Design review of the part built by this model. Coordinates are the model's own, in mm. A direction names the side the tool comes from. Round coordinates to 2 decimals unless told otherwise and drop trailing zeros. Order: outer loops, then holes, each group sorted by start corner. A loop starts at its lowest first (then second) coordinate and runs counter-clockwise, first axis right, second up. Notation, with made-up numbers: (74.5, -40) - (119.5, -40) arc R18 ccw to (119.5, -14) - close; hole circle Ø6 at (5, 77). An arc over 180 degrees is marked (long way). Answer as a JSON object with one key per item and string values. Group by question number.
from build123d import *

# Parameters (mm, degrees)
SKETCH3_W                      = 207
SKETCH3_H                      = 195
BASE_FLANGE1_DEPTH             = 2
EDGE_FLANGE1_STRIP_W           = 9.4732
EDGE_FLANGE1_STRIP_H           = 2
EDGE_FLANGE1_STRIP_CUT_DEPTH   = 207
EDGE_FLANGE1_STRIP_2_W         = 9.4732
EDGE_FLANGE1_STRIP_2_H         = 2
EDGE_FLANGE1_STRIP_CUT_2_DEPTH = 207
EDGE_FLANGE1_DEPTH             = 207
EDGE_FLANGE1_BEND_DEPTH        = 207
SKETCH14_R                     = 68.5
CUT_EXTRUDE1_DEPTH             = 2
EDGE_FLANGE2_DEPTH             = 207
EDGE_FLANGE2_BEND_DEPTH        = 207


# Sheet-metal steps are written as plain solids
with BuildPart() as part:
    # Sketch3 → Base-Flange1 (new body)
    with BuildSketch(Plane(origin=(0, 0, 0), x_dir=(1, 0, 0), z_dir=(0, 1, 0))):
        with Locations((-1.354892482, -0.135489248)):
            Rectangle(SKETCH3_W, SKETCH3_H)
    extrude(amount=-BASE_FLANGE1_DEPTH)

    # Edge-Flange1 strip (across the edge) → Edge-Flange1 strip cut (cut)
    with BuildSketch(Plane(origin=(102.145107518, -2, 97.635489248), x_dir=(0, 0, -1), z_dir=(-1, 0, 0))):
        with Locations((-2, -1)):
            Rectangle(EDGE_FLANGE1_STRIP_W, EDGE_FLANGE1_STRIP_H)
    extrude(amount=EDGE_FLANGE1_STRIP_CUT_DEPTH, mode=Mode.SUBTRACT)

    # Edge-Flange1 strip 2 (across the edge) → Edge-Flange1 strip cut 2 (cut)
    with BuildSketch(Plane(origin=(-104.854892482, -2, -97.364510752), x_dir=(0, 0, 1), z_dir=(1, 0, 0))):
        with Locations((-2, -1)):
            Rectangle(EDGE_FLANGE1_STRIP_2_W, EDGE_FLANGE1_STRIP_2_H)
    extrude(amount=EDGE_FLANGE1_STRIP_CUT_2_DEPTH, mode=Mode.SUBTRACT)

    # Edge-Flange1 section (across the edge) → Edge-Flange1 (add)
    with BuildSketch(Plane(origin=(102.145107518, -2, 97.635489248), x_dir=(0, 0, -1), z_dir=(-1, 0, 0))):
        with BuildLine():
            Line((0, 0.7366), (0, 23))
            Line((0, 23), (2, 23))
            Line((2, 23), (2, 0.7366))
            ThreePointArc((2, 0.7366), (2.215745145, 0.215745145), (2.7366, 0))
            Line((2.7366, 0), (2.7366, -2))
            ThreePointArc((2.7366, -2), (0.801531583, -1.198468417), (0, 0.7366))
        make_face()
    extrude(amount=EDGE_FLANGE1_DEPTH)

    # Edge-Flange1 section 2 (across the edge) → Edge-Flange1 bend (add)
    with BuildSketch(Plane(origin=(-104.854892482, -2, -97.364510752), x_dir=(0, 0, 1), z_dir=(1, 0, 0))):
        with BuildLine():
            Line((0, 0.7366), (0, 23))
            Line((0, 23), (2, 23))
            Line((2, 23), (2, 0.7366))
            ThreePointArc((2, 0.7366), (2.215745145, 0.215745145), (2.7366, 0))
            Line((2.7366, 0), (2.7366, -2))
            ThreePointArc((2.7366, -2), (0.801531583, -1.198468417), (0, 0.7366))
        make_face()
    extrude(amount=EDGE_FLANGE1_BEND_DEPTH)

    # Sketch14 → Cut-Extrude1 (cut)
    with BuildSketch(Plane(origin=(0, 0, 0), x_dir=(1, 0, 0), z_dir=(0, 1, 0))):
        with Locations(Location((-1.354892482, -0.135489248, 0), (0, 0, 270))):
            Circle(SKETCH14_R)
    extrude(amount=-CUT_EXTRUDE1_DEPTH, mode=Mode.SUBTRACT)

    # Edge-Flange2 section (across the edge) → Edge-Flange2 (add)
    with BuildSketch(Plane(origin=(102.145107518, -25.7366, 95.635489248), x_dir=(0, 1, 0), z_dir=(-1, 0, 0))):
        with BuildLine():
            Line((-2, 0.7366), (-2, 14))
            Line((-2, 14), (0, 14))
            Line((0, 14), (0, 0.7366))
            ThreePointArc((0, 0.7366), (0.215745145, 0.215745145), (0.7366, 0))
            Line((0.7366, 0), (0.7366, -2))
            ThreePointArc((0.7366, -2), (-1.198468417, -1.198468417), (-2, 0.7366))
        make_face()
    extrude(amount=EDGE_FLANGE2_DEPTH)

    # Edge-Flange2 section 2 (across the edge) → Edge-Flange2 bend (add)
    with BuildSketch(Plane(origin=(-104.854892482, -25.7366, -95.364510752), x_dir=(0, 1, 0), z_dir=(1, 0, 0))):
        with BuildLine():
            Line((-2, 0.7366), (-2, 14))
            Line((-2, 14), (0, 14))
            Line((0, 14), (0, 0.7366))
            ThreePointArc((0, 0.7366), (0.215745145, 0.215745145), (0.7366, 0))
            Line((0.7366, 0), (0.7366, -2))
            ThreePointArc((0.7366, -2), (-1.198468417, -1.198468417), (-2, 0.7366))
        make_face()
    extrude(amount=EDGE_FLANGE2_BEND_DEPTH)


solid = part.part
1. Take a section at C-C, the plane z = -46. Give the boundary of the cut face in (x, y).
2. Clearance check with flat-ended pins moving along their axes: P1, Ø12, axis at x = -75.5, z = -71, coming from the -Y side; P2, Ø10.5, axis at x = 30, z = 89, coming from the +Y side; P3, Ø2, axis at x = 14.5, y = -26.5, coming from the -Z side; P4, Ø0.6, axis at x = 35, y = -26.5, coming from the +Z side. State where each tip first meets the part, or that it passes through.
3. Tool access review of faces 5 (the flat face through (0, -27.737, 88)), 6 (the flat face through (-3, -25.737, -88)): name each direction out of +Z, -Z, +X, -X, +Y, -Y from which nothing blocks a thin tool from reaching the whole face with its end or side.
4. Take a section at D-D, the plane x = -81.5. Give the boundary of the cut face in (y, z).
5. Take a section at A-A, the plane y = -19.5. Give the boundary of the cut face in (x, z).
6. To check wall thickness, follow line 1 (Y direction, x = -25, z = -84.5); line 2 (Z direction, x = -40.5, y = -25.25); line 3 (Z direction, x = 6.5, y = -8.25). State the ranges of each line that lie inside material, in increasing order. Write a range as from..to.
7. Mouldability with a two-part tool opening along X and no side actions: class faces 1 (the flat face through (0, -14, 95.635)), 2 (the cylindrical face through (19.221, -0.986, 65.472)), 3 (the flat face through (-104.855, -1, 1)), 4 (the flat face through (102.145, -1, 1)) as pulls with the +X half, pulls with the -X half, needs draft (parallel to the pull), parting line crosses it, or undercut.
8. Take a section at B-B, the plane x = -19. Give the boundary of the cut face in (y, z), then the cut area to 3 significant figures.
Response values:
{
 "1": {"outline": "(-104.85, -2) - (-51.99, -2) - (-51.99, 0) - (-104.85, 0) - close; (49.28, -2) - (102.15, -2) - (102.15, 0) - (49.28, 0) - close"},
 "2": {"P1": "y = -2", "P2": "y = 0", "P3": "z = -97.32", "P4": "z = 97.36"},
 "3": {"face 5": "+Z, -Z, +X, -X, -Y", "face 6": "+X, -X"},
 "4": {"outline": "(-27.74, -94.63) arc R2.74 ccw to (-25, -97.36) - (-2.74, -97.36) arc R2.74 ccw to (0, -94.63) - (0, 94.9) arc R2.74 ccw to (-2.74, 97.64) - (-25, 97.64) arc R2.74 ccw to (-27.74, 94.9) - (-27.74, 81.64) - (-25.74, 81.64) - (-25.74, 94.9) arc R0.74 cw to (-25, 95.64) - (-2.74, 95.64) arc R0.74 cw to (-2, 94.9) - (-2, -94.63) arc R0.74 cw to (-2.74, -95.36) - (-25, -95.36) arc R0.74 cw to (-25.74, -94.63) - (-25.74, -81.36) - (-27.74, -81.36) - close"},
 "5": {"outline": "(-104.85, -97.36) - (102.15, -97.36) - (102.15, -95.36) - (-104.85, -95.36) - close; (-104.85, 95.64) - (102.15, 95.64) - (102.15, 97.64) - (-104.85, 97.64) - close"},
 "6": {"line 1": "-27.74..-25.74, -2..0", "line 2": "-97.35..-95.32, 95.59..97.62", "line 3": "-97.36..-95.36, 95.64..97.64"},
 "7": {"face 1": "needs draft", "face 2": "undercut", "face 3": "pulls with the -X half", "face 4": "pulls with the +X half"},
 "8": {"outline": "(-27.74, -94.63) arc R2.74 ccw to (-25, -97.36) - (-2.74, -97.36) arc R2.74 ccw to (0, -94.63) - (0, -66.05) - (-2, -66.05) - (-2, -94.63) arc R0.74 cw to (-2.74, -95.36) - (-25, -95.36) arc R0.74 cw to (-25.74, -94.63) - (-25.74, -81.36) - (-27.74, -81.36) - close; (-27.74, 81.64) - (-25.74, 81.64) - (-25.74, 94.9) arc R0.74 cw to (-25, 95.64) - (-2.74, 95.64) arc R0.74 cw to (-2, 94.9) - (-2, 66.32) - (0, 66.32) - (0, 94.9) arc R2.74 ccw to (-2.74, 97.64) - (-25, 97.64) arc R2.74 ccw to (-27.74, 94.9) - close", "area": "278 mm2"}
}
